Design review of the part built by this model. Coordinates are the model's own, in mm. Face numbers are marked on the shaded views. A direction names the side the tool comes from. Round coordinates to 2 decimals unless told otherwise and drop trailing zeros. Order: outer loops, then holes, each group sorted by start corner. A loop starts at its lowest first (then second) coordinate and runs counter-clockwise, first axis right, second up. Notation, with made-up numbers: M -32.75,81.5 L 16.25,81.5 A28 ccw 16.25,108.5 Z; hole C 8,4 d2. An arc over 180 degrees is marked long. Use a Markdown table: item, result. Add a question column.
(1) The part is to be moulded in two halves that separate along Y. For the marked faces 1, 2 and 3, say which applies: released by +Y, released by -Y, zero draft, split by the parting line, or undercut.
(2) Take a section at B-B (x = 10). Write out the cut boundary in (y, z), then the cut area to 3 significant figures.
(3) Take a section at A-A (y = -0.5). Write out the cut boundary in (x, z), then the cut area to 3 significant figures.
(4) To check wall thickness, follow probe 1 along Y at (x, z) = (22.65, 0); probe 2 along Y at (x, z) = (24.65, 0); probe 3 along Z at (x, y) = (7, -4.25). State the ranges of each line that lie inside material, in increasing order. Write a range as from..to.
(5) For pin 1 (2 mm diameter, centred on x = 11.5, z = 5.5, fed in from -Y); pin 2 (1.4 mm diameter, centred on y = 6.5, z = 0, fed in from -X); pin 3 (4 mm diameter, centred on x = 21, y = -1.5, fed in from +Z); pin 4 (1.5 mm diameter, centred on x = 14.5, z = -1, fed in from -Y), all flat-tipped, find the tip position at first contact; note any pin that passes through.
(6) Take a section at C-C (z = -0.25). Write out the cut boundary in (x, y), then the cut area to 3 significant figures.
(7) Machinability: for the marked faces 4, 5, 6 and 7, which of the approach directions +Z, -Z, +X, -X, +Y, -Y give a long, thin tool a straight path to every point of the face, cutting with its end or side? Answer none if there is none.
(8) Take a section at D-D (z = -4.25). Write out the cut boundary in (x, y).
Autodesk Inventor part; units mm, degrees
ref_plane "Work Plane1" through (21, 10, -5.75) normal (0.9701266, 0.2425992, 0) x (0, 0, 1)
ref_plane "Work Plane2" through (28.427, 0, 0) normal (-1, 0, 0) x (0, 0, 1)
ref_plane "YZ Plane" through (0, 0, 0) normal (1, 0, 0) x (0, 1, 0)
sketch "Sketch1" plane through (0, 0, 0) normal (1, 0, 0) x (0, 1, 0)
  line L0 (-10, 5.75) -> (10, 5.75)
  line L1 (10, 5.75) -> (10, -5.75)
  line L2 (10, -5.75) -> (-10, -5.75)
  line L3 (-10, -5.75) -> (-10, 5.75)
  line L4 (-10, 5.75) -> (10, -5.75) construction
  line L5 (10, 5.75) -> (-10, -5.75) construction
  point P0 (0, 0)
  dimension "d0" = 20
  dimension "d1" = 11.5
extrude "Extrusion1" add sketch "Sketch1" along normal blind 21
ref_plane "Work Plane1" through (21, 10, -5.75) normal (0.9701266, 0.2425992, 0) x (0, 0, 1)
sketch "Sketch2" plane through (0, 10, 5.75) normal (0, 1, 0) x (1, 0, 0)
  line L0 (7.75, 5.1) -> (2.25, 5.1)
  line L1 (2.25, 5.1) -> (2.25, 6.4)
  line L2 (2.25, 6.4) -> (7.75, 6.4)
  line L3 (7.75, 6.4) -> (7.75, 5.1)
  line L4 (7.75, 5.1) -> (2.25, 6.4) construction
  line L5 (2.25, 5.1) -> (7.75, 6.4) construction
  line L6 (7.25, 5.1) -> (2.75, 5.1)
  line L7 (2.75, 5.1) -> (2.75, 6.4)
  line L8 (2.75, 6.4) -> (7.25, 6.4)
  line L9 (7.25, 6.4) -> (7.25, 5.1)
  line L10 (7.25, 5.1) -> (2.75, 6.4) construction
  line L11 (2.75, 5.1) -> (7.25, 6.4) construction
  line L12 (0, 11.5) -> (0, 0) construction
  point P0 (0, 5.75)
  point P1 (5, 5.75)
  point P2 (5, 5.75)
  point P3 (7.25, 5.1)
  point P4 (2.75, 5.1)
  point P5 (0, 5.75)
  dimension "d4" = 5.5
  dimension "d5" = 1.3
  dimension "d6" = 4.5
  dimension "d20" = 5
extrude "Extrusion2" cut sketch "Sketch2" against normal blind 10
extrude "Extrusion3" cut sketch "Sketch2" against normal blind 14 contours L0 L7 L2 L9
fillet "Fillet1" radius 3 4 edges at (0, 0, 5.75) (10.5, -10, 5.75) (10.5, -10, -5.75) (0, 0, -5.75)
fillet "Fillet2" radius 7 3 edges at (0.8787, -9.1213, -4.8713) (0.8787, -9.1213, 4.8713) (0, -10, 0)
sketch "Sketch4" plane through (21, 0, 0) normal (1, 0, 0) x (0, 0, -1)
  arc A0 (2.75, -10) -> (5.75, -7) centre (2.75, -7) ccw
  line L0 (5.75, -7) -> (5.75, 10)
  line L1 (5.75, 10) -> (-5.75, 10)
  line L2 (-5.75, 10) -> (-5.75, -7)
  arc A1 (-5.75, -7) -> (-2.75, -10) centre (-2.75, -7) ccw
  line L3 (-2.75, -10) -> (2.75, -10)
  point P0 (0, 0)
extrude "Extrusion5" add sketch "Sketch4" along normal up to surface surface through (21, 10, -5.75) normal (0.9701266, 0.2425992, 0)
sketch "Sketch6" plane through (21, 10, 5.75) normal (0.9701266, 0.2425992, 0) x (0, 0, -1)
  line L0 (11.5, 0) -> (11.5, -17.5235)
  line L1 (11.5, 0) -> (0, 0)
  line L2 (0, -17.5235) -> (0, 0)
  line L3 (8.5, -20.6159) -> (3, -20.6159)
  line L4 (-1.5, 0) -> (13, 0)
  line L5 (13, 0) -> (13, -18.7739)
  line L6 (9.158, -22.6159) -> (2.342, -22.6159)
  line L7 (-1.5, -18.7739) -> (-1.5, 0)
  arc A0 (-1.5, -18.7739) -> (2.342, -22.6159) centre (2.342, -18.7739) ccw
  arc A1 (9.158, -22.6159) -> (13, -18.7739) centre (9.158, -18.7739) ccw
  point P0 (5.75, -4.6067)
  dimension "d21" = 1.5
  dimension "d22" = 1.5
  dimension "d23" = 2
  dimension "d24" = 3.842
extrude "Extrusion6" add sketch "Sketch6" along normal blind 2
sketch "Sketch7" plane through (0, 0, 0) normal (-1, 0, 0) x (0, 0, 1)
  line L0 (7.25, 10.4852) -> (7.25, -7.7278) construction
  line L1 (-7.6184, 10) -> (7.25, 10)
  line L2 (7.25, 10) -> (7.25, 10.4852)
  line L3 (7.25, 10.4852) -> (-7.6184, 10.4852)
  line L4 (-7.6184, 10.4852) -> (-7.6184, 10)
  line L5 (3.408, -11.4551) -> (-3.408, -11.4551) construction
  line L6 (-3.408, -11.4551) -> (7.25, -11.4551)
  line L7 (7.25, -11.4551) -> (7.25, -13.162)
  line L8 (7.25, -13.162) -> (-3.408, -13.162)
  line L9 (-3.408, -13.162) -> (-3.408, -11.4551)
  line L10 (-3.408, -11.4551) -> (-7.4388, -11.4551)
  line L11 (-7.4388, -11.4551) -> (-7.4388, -13.1256)
  line L12 (-7.4388, -13.1256) -> (-3.408, -13.1256)
  line L13 (-3.408, -13.1256) -> (-3.408, -11.4551)
  point P0 (0, 0)
  point P1 (-2.75, 10)
extrude "Extrusion7" cut sketch "Sketch7" against normal through all
ref_plane "Work Plane2" through (28.427, 0, 0) normal (-1, 0, 0) x (0, 0, 1)
sketch "Sketch8" plane through (28.427, 0, 0) normal (-1, 0, 0) x (0, 0, 1)
  circle A0 centre (0, 1.5449) radius 2.75
  circle A1 centre (0, -6.4551) radius 2.75
  line L0 (3.408, -11.4551) -> (-3.408, -11.4551) construction
  point P0 (0, 0)
  dimension "d30" = 5.5
  dimension "d31" = 5.5
  dimension "d36" = 8
  dimension "d37" = 5
extrude "Extrusion8" cut sketch "Sketch8" along normal blind 5.5 contours A1
extrude "Extrusion9" cut sketch "Sketch8" along normal blind 7.5 contours A0
properties part number "buton" material "PBT Plastic"
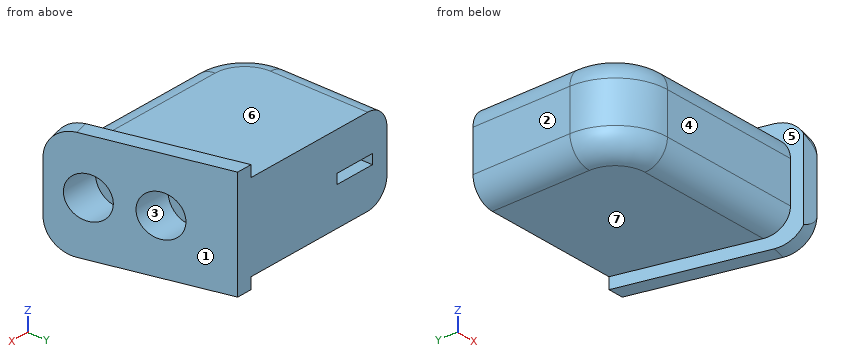
Verdict:
| question | item | result |
|---|---|---|
| 1 | face 1 | released by +Y |
| 1 | face 2 | zero draft |
| 1 | face 3 | undercut |
| 2 | outline | M -10,-2.75 A3 ccw -7,-5.75 L 10,-5.75 L 10,5.75 L -7,5.75 A3 ccw -10,2.75 Z |
| 2 | area | 226 mm^2 |
| 3 | outline | M 0,-2.75 A3 ccw 3,-5.75 L 23.63,-5.75 L 23.63,-7.25 L 25.69,-7.25 L 25.69,-1.84 L 20.93,-1.84 L 20.93,1.84 L 25.69,1.84 L 25.69,7.25 L 23.63,7.25 L 23.63,5.75 L 3,5.75 A3 ccw 0,2.75 Z; hole M 2.75,-0.65 L 7.25,-0.65 L 7.25,0.65 L 2.75,0.65 Z |
| 3 | area | 274 mm^2 |
| 4 | probe 1 | y = -10..-1.21, 4.29..10 |
| 4 | probe 2 | y = -10..-9.21, -3.71..-1.21 |
| 4 | probe 3 | z = -5.75..5.75 |
| 5 | pin 1 | stops at y = -9.44 |
| 5 | pin 2 | stops at x = 0 |
| 5 | pin 3 | stops at z = 5.75 |
| 5 | pin 4 | stops at y = -10 |
| 6 | outline | M 0,-3 A7 ccw 7,-10 L 26,-10 L 26.37,-11.46 L 28.43,-11.46 L 27.86,-9.19 L 22.93,-9.19 L 22.93,-3.72 L 26.49,-3.72 L 25.86,-1.19 L 20.93,-1.19 L 20.93,4.28 L 24.49,4.28 L 23.06,10 L 7.75,10 L 7.75,0 L 7.25,0 L 7.25,-4 L 2.75,-4 L 2.75,0 L 2.25,0 L 2.25,10 L 0,10 Z |
| 6 | area | 384 mm^2 |
| 7 | face 4 | +Z, -Z, -X, -Y |
| 7 | face 5 | -X, -Y |
| 7 | face 6 | +Z, -X, -Y |
| 7 | face 7 | -Z, -X, -Y |
| 8 | outline | M 0.4,-3 A6.6 ccw 7,-9.6 L 25.9,-9.6 L 26.37,-11.46 L 28.04,-11.46 L 28.4,-11.36 L 23.06,10 L 0.4,10 Z |
